Model file for the job. Use its own axes, mm. A direction names the side the tool comes from. Coordinates: 2 decimals unless noted, no trailing zeros. Loops run counter-clockwise (first coordinate to the right, second up) from the corner with the lowest first, then second, coordinate; pieces in that order, holes last.
Autodesk Fusion 360 part; units mm, degrees
sketch "スケッチ2" plane through (0, 0, 0) normal (0, 0, 1) x (1, 0, 0)
  line L0 (-18, 16) -> (18, 16)
  line L1 (18, 16) -> (18, -16)
  line L2 (18, -16) -> (-18, -16)
  line L3 (-18, -16) -> (-18, 16)
  point P0 (18, 0)
  dimension "d8" = 32
  dimension "d9" = 18
  dimension "d10" = 18
extrude "押し出し2" add sketch "スケッチ2" along normal blind 8
sketch "スケッチ3" plane through (0, 0, 8) normal (0, 0, 1) x (-1, 0, 0)
  line L0 (18, 16) -> (-18, 16)
  line L1 (-18, 16) -> (-18, -16)
  line L2 (-18, -16) -> (18, -16)
  line L3 (18, -16) -> (18, 16)
  circle A0 centre (0, 0) radius 10
  dimension "d13" = 20
extrude "押し出し3" add sketch "スケッチ3" along normal blind 5 contours A0
sketch "スケッチ4" plane through (0, 0, 13) normal (0, 0, 1) x (-1, 0, 0)
  circle A0 centre (0, 0) radius 10
  circle A1 centre (0, 0) radius 7
  line L0 (7, 0) -> (-7, 0)
  line L1 (0, -7) -> (0, 7)
  dimension "d16" = 14
hole "穴2" at (-7, 0, 13) at (0, 7, 13) at (7, 0, 13) at (0, -7, 13) direction (0, 0, -1) diameter 3.2 end through all
sketch "スケッチ5" plane through (0, -16, 0) normal (0, -1, 0) x (1, 0, 0)
  line L0 (-18, 0) -> (18, 0)
  line L1 (18, 0) -> (18, 8)
  line L2 (18, 8) -> (-18, 8)
  line L3 (-18, 8) -> (-18, 0)
  line L4 (-13, 4) -> (13, 4)
  dimension "d21" = 5
  dimension "d23" = 4
  dimension "d24" = 5
hole "穴3" at (-13, -16, 4) at (13, -16, 4) direction (0, 1, 0) diameter 3 depth 10 tip angle 118
sketch "スケッチ6" plane through (0, 16, 0) normal (0, 1, 0) x (-1, 0, 0)
  line L0 (-18, 0) -> (18, 0)
  line L1 (18, 0) -> (18, 8)
  line L2 (18, 8) -> (-18, 8)
  line L3 (-18, 8) -> (-18, 0)
  line L4 (-13, 4) -> (13, 4)
  dimension "d28" = 4
  dimension "d29" = 5
  dimension "d30" = 5
hole "穴4" at (13, 16, 4) at (-13, 16, 4) direction (0, -1, 0) diameter 3 depth 10 tip angle 118
thread "ねじ2"
sketch "スケッチ7" plane through (0, 0, 0) normal (0, 0, -1) x (1, 0, 0)
  circle A0 centre (7, 0) radius 1.6
  circle A1 centre (-7, 0) radius 1.6
  circle A2 centre (0, -7) radius 1.6
  circle A3 centre (0, 7) radius 1.6
  line L0 (18, 16) -> (-18, 16)
  line L1 (-18, 16) -> (-18, -16)
  line L2 (-18, -16) -> (18, -16)
  line L3 (18, -16) -> (18, 16)
  circle A4 centre (0, 0) radius 11
  dimension "d34" = 22
extrude "押し出し4" cut sketch "スケッチ7" against normal blind 2 contours A4
hole "穴5" at (0, 0, 13) direction (0, 0, -1) diameter 8 end through all
Q1. Flat gauge pins, fed straight in: P1, Ø5, axis at x = 7, y = 0, coming from the +Z side; P2, Ø2, axis at x = 6.5, z = 11, coming from the -Y side; P3, Ø6.5, axis at x = 0, y = 0, coming from the -Z side; P4, Ø2.5, axis at x = -13, z = 4, coming from the +Y side. Where does each tip first touch, or does it go through?
Answers:
P1: stops at z = 13
P2: stops at y = -8.35
P3: passes through
P4: stops at y = 5.85
Q2. Which spindle directions (+Z, -Z, +X, -X, +Y, -Y) get a long thin tool onto all of the face, cutting with end or side? Do faces 4 (the flat face through (0, 11, 8)), 5 (the cylindrical face through (13.575, -10.93, 2.614)), 6 (the flat face through (0, 5, 2)). Say none if no direction does.
Answers:
face 4: +Z
face 5: -Y
face 6: -Z
Q3. Slice it at D-D (y = 2.5). List the corners of the cut face in (x, z).
Answers:
outline: (-18, 0) - (-10.71, 0) - (-10.71, 2) - (-3.12, 2) - (-3.12, 13) - (-9.68, 13) - (-9.68, 8) - (-18, 8) - close; (3.12, 2) - (10.71, 2) - (10.71, 0) - (18, 0) - (18, 8) - (9.68, 8) - (9.68, 13) - (3.12, 13) - close
Q4. Slice it at C-C (y = 7). List the corners of the cut face in (x, z).
Answers:
outline: (-18, 0) - (-8.49, 0) - (-8.49, 2) - (-1.6, 2) - (-1.6, 13) - (-7.14, 13) - (-7.14, 8) - (-18, 8) - close; (1.6, 2) - (8.49, 2) - (8.49, 0) - (18, 0) - (18, 8) - (7.14, 8) - (7.14, 13) - (1.6, 13) - close; hole circle Ø3 at (-13, 4); hole circle Ø3 at (13, 4)
Q5. Drill centre lines: line 1 (Y direction, x = 0, z = 6.5); line 2 (Y direction, x = 0, z = 1.35); line 3 (X direction, y = 0, z = 5.25). Where is each one in solid material? Low to high.
Answers:
line 1: y = -16 to -8.6, -5.4 to -4, 4 to 5.4, 8.6 to 16
line 2: y = -16 to -11, 11 to 16
line 3: x = -18 to -8.6, -5.4 to -4, 4 to 5.4, 8.6 to 18
Q6. Slice it at B-B (z = 6.5). List the corners of the cut face in (x, y).
Answers:
outline: (-18, -16) - (18, -16) - (18, 16) - (-18, 16) - close; hole circle Ø3.2 at (-7, 0); hole circle Ø8 at (0, 0); hole circle Ø3.2 at (0, -7); hole circle Ø3.2 at (0, 7); hole circle Ø3.2 at (7, 0)
Q7. Slice it at A-A (x = 0). List the corners of the cut face in (y, z).
Answers:
outline: (-16, 0) - (-11, 0) - (-11, 2) - (-8.6, 2) - (-8.6, 13) - (-10, 13) - (-10, 8) - (-16, 8) - close; (-5.4, 2) - (-4, 2) - (-4, 13) - (-5.4, 13) - close; (4, 2) - (5.4, 2) - (5.4, 13) - (4, 13) - close; (8.6, 2) - (11, 2) - (11, 0) - (16, 0) - (16, 8) - (10, 8) - (10, 13) - (8.6, 13) - close
Q8. Mould opens along X. For faces 1 (the flat face through (0, 16, 4)), 2 (the cylindrical face through (-12.425, -10.93, 2.614)), 3 (the flat face through (18, 0, 4)) say: +X half, -X half, draft (parallel to the pull), parting line (faces both ways), or undercut.
Answers:
face 1: draft
face 2: undercut
face 3: +X half
